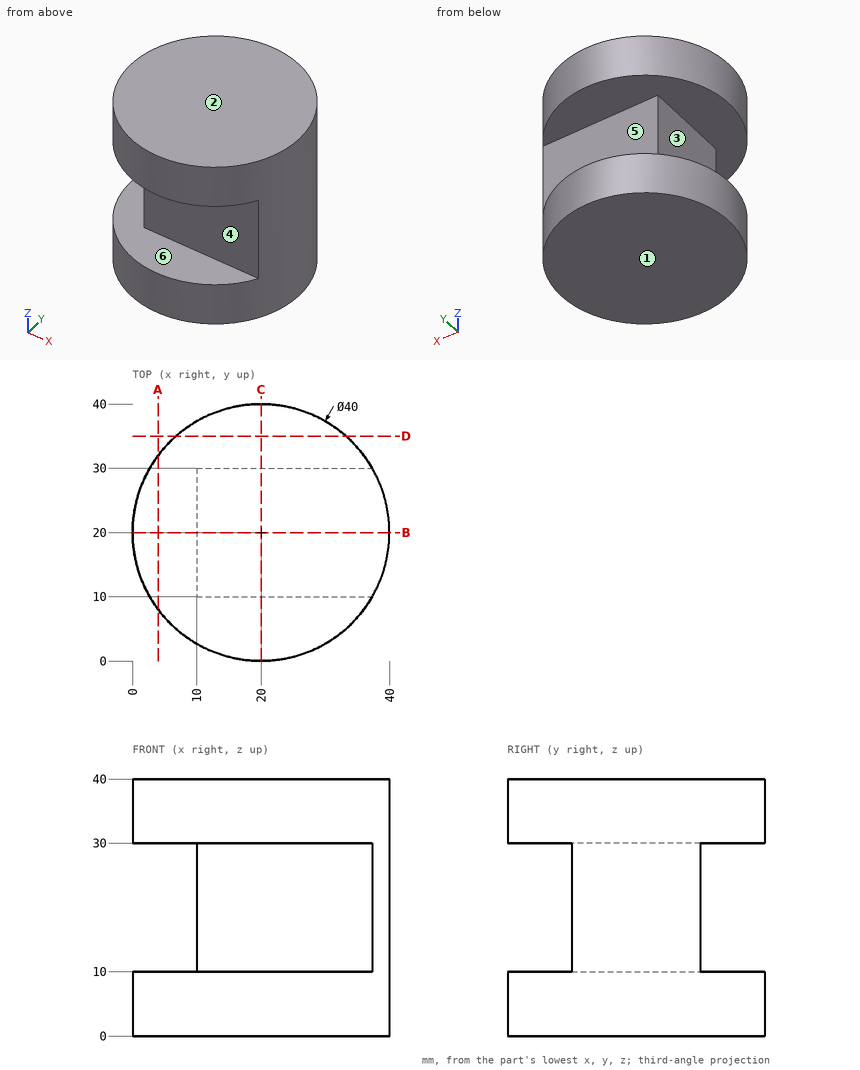
Can you work these out from the drawing? Everything is in mm from the part's minimum corner. A direction names the side the tool comes from. Round coordinates to 2 decimals unless told otherwise and drop trailing zeros. Order: outer loops, then holes, each group sorted by start corner. A loop starts at its lowest first (then second) coordinate and runs counter-clockwise, first axis right, second up.
(1) If we section it at A-A (x = 4): Please give me the cut outline in (y, z), plus the area to 3 significant figures.
Results are:
outline: (8, 0) - (32, 0) - (32, 10) - (8, 10) - close; (8, 30) - (32, 30) - (32, 40) - (8, 40) - close
area: 480 mm2
(2) If we section it at B-B (y = 20): Please give me the cut outline in (x, z), plus the area to 3 significant figures.
Results are:
outline: (0, 0) - (40, 0) - (40, 40) - (0, 40) - (0, 30) - (10, 30) - (10, 10) - (0, 10) - close
area: 1,400 mm2
(3) If we section it at C-C (x = 20): Please give me the cut outline in (y, z), plus the area to 3 significant figures.
Results are:
outline: (0, 0) - (40, 0) - (40, 10) - (30, 10) - (30, 30) - (40, 30) - (40, 40) - (0, 40) - (0, 30) - (10, 30) - (10, 10) - (0, 10) - close
area: 1,200 mm2
(4) On a 3-axis mill with a long thin cutter (end or side, diameter ignored), from which of +Z, -Z, +X, -X, +Y, -Y can I reach the whole of each face in a straight line? I mean the marked faces 4, 5 and 6. Say none if no direction works.
Results are:
face 4: +X, -X, -Y
face 5: +X, -X, +Y
face 6: -X
(5) If we section it at D-D (y = 35): Please give me the cut outline in (x, z), plus the area to 3 significant figures.
Results are:
outline: (6.77, 0) - (33.23, 0) - (33.23, 10) - (6.77, 10) - close; (6.77, 30) - (33.23, 30) - (33.23, 40) - (6.77, 40) - close
area: 529 mm2
(6) We'd pull the mould along Z, two halves only. Please class the marked faces 1, 2 and 3: +Z half, -Z half, draft (parallel to the pull), parting line (faces both ways), or undercut.
Results are:
face 1: -Z half
face 2: +Z half
face 3: undercut
(7) I'm going to push flat-ended pins straight in: pin 1 (12 mm diameter, centred on y = 19.5, z = 14.5, fed in from +X); pin 2 (3 mm diameter, centred on x = 16.5, z = 6, fed in from -Y); pin 3 (6 mm diameter, centred on y = 19, z = 17, fed in from -X); pin 4 (6 mm diameter, centred on x = 7.5, z = 4.5, fed in from +Y). Where does each tip first touch, or does it pass through?
Results are:
pin 1: stops at x = 40
pin 2: stops at y = 0.1
pin 3: stops at x = 10
pin 4: stops at y = 37.6
(8) If I drill on L1, parallel to Z at x = 5.5, y = 7.5; L2, parallel to Y at x = 24, z = 17; L3, parallel to Y at x = 37.5, z = 36.5, over which ranges is the centre line in solid material (lowest first)?
Results are:
L1: z = 0 to 10, 30 to 40
L2: y = 10 to 30
L3: y = 10.32 to 29.68
